```python
from build123d import *

# Parameters (mm, degrees)
CROQUIS1_W                 = 45
CROQUIS1_H                 = 45
SALIENTE_EXTRUIR1_DEPTH    = 300
CROQUIS4_W                 = 18
CROQUIS4_H                 = 34
CORTAR_EXTRUIR2_DEPTH      = 46
CROQUIS8_W                 = 35
CROQUIS8_H                 = 35
CORTAR_EXTRUIR3_DEPTH      = 301
CROQUIS9_W                 = 35
CROQUIS9_H                 = 21.174410022
CORTAR_EXTRUIR4_DEPTH      = 10
CROQUIS10_R                = 1
CORTAR_EXTRUIR5_DEPTH      = 10
CROQUIS11_W                = 45
CROQUIS11_H                = 26.387879272
CORTAR_EXTRUIR6_DEPTH      = 46
CROQUIS13_W                = 45
CROQUIS13_H                = 100
CORTAR_EXTRUIR7_DEPTH      = 23.5
CORTAR_EXTRUIR7_DEPTH_BACK = 23.5
CROQUIS14_W                = 55
CROQUIS14_H                = 55
SALIENTE_EXTRUIR2_DEPTH    = 5
CROQUIS16_R                = 1
CORTAR_EXTRUIR8_DEPTH      = 1
CORTAR_EXTRUIR8_DEPTH_BACK = 179.612120728
CROQUIS17_R                = 2.5
CROQUIS17_R_2              = 2.03
CROQUIS17_R_3              = 1.793308219
CORTAR_EXTRUIR9_DEPTH      = 6
CORTAR_EXTRUIR9_DEPTH_BACK = 51


with BuildPart() as part:
    # Croquis1 → Saliente-Extruir1 (new body)
    with BuildSketch(Plane(origin=(0, 0, 0), x_dir=(1, 0, 0), z_dir=(0, 1, 0))):
        Rectangle(CROQUIS1_W, CROQUIS1_H)
    extrude(amount=SALIENTE_EXTRUIR1_DEPTH)

    # Croquis4 → Cortar-Extruir2 (cut, through all)
    with BuildSketch(Plane.ZY.offset(22.5)):
        with Locations((13.5, 17)):
            Rectangle(CROQUIS4_W, CROQUIS4_H)
    extrude(amount=-CORTAR_EXTRUIR2_DEPTH, mode=Mode.SUBTRACT)

    # Croquis8 → Cortar-Extruir3 (cut, through all)
    with BuildSketch(Plane(origin=(0, 300, 0), x_dir=(1, 0, 0), z_dir=(0, 1, 0))):
        Rectangle(CROQUIS8_W, CROQUIS8_H)
    extrude(amount=-CORTAR_EXTRUIR3_DEPTH, mode=Mode.SUBTRACT)

    # Croquis9 → Cortar-Extruir4 (cut)
    with BuildSketch(Plane(origin=(0, 0, -22.5), x_dir=(-1, 0, 0), z_dir=(0, 0, -1))):
        with Locations((0, 260)):
            Rectangle(CROQUIS9_W, CROQUIS9_H)
    extrude(amount=-CORTAR_EXTRUIR4_DEPTH, mode=Mode.SUBTRACT)

    # Croquis10 → Cortar-Extruir5 (cut)
    with BuildSketch(Plane.XY.offset(22.5)):
        with Locations((0, 260)):
            Circle(CROQUIS10_R)
    extrude(amount=-CORTAR_EXTRUIR5_DEPTH, mode=Mode.SUBTRACT)

    # Croquis11 → Cortar-Extruir6 (cut, through all)
    with BuildSketch(Plane.XY.offset(22.5)):
        with Locations((0, 286.806060364)):
            Rectangle(CROQUIS11_W, CROQUIS11_H)
    extrude(amount=-CORTAR_EXTRUIR6_DEPTH, mode=Mode.SUBTRACT)

    # Croquis13 → Cortar-Extruir7 (cut, two sides)
    with BuildSketch(Plane(origin=(0, 0, 0), x_dir=(0, 0, -1), z_dir=(1, 0, 0))) as cortar_extruir7_sk:
        with Locations((0, 50)):
            Rectangle(CROQUIS13_W, CROQUIS13_H)
    extrude(amount=CORTAR_EXTRUIR7_DEPTH, mode=Mode.SUBTRACT)
    extrude(cortar_extruir7_sk.sketch, amount=-CORTAR_EXTRUIR7_DEPTH_BACK, mode=Mode.SUBTRACT)

    # Croquis14 → Saliente-Extruir2 (add)
    with BuildSketch(Plane.XZ.offset(-100)):
        Rectangle(CROQUIS14_W, CROQUIS14_H)
    extrude(amount=SALIENTE_EXTRUIR2_DEPTH)

    # Croquis16 → Cortar-Extruir8 (cut, two sides)
    with BuildSketch(Plane.XZ.offset(-95)) as cortar_extruir8_sk:
        with Locations((25, 25)):
            Circle(CROQUIS16_R)
        with Locations((-25, 25)):
            Circle(CROQUIS16_R)
        with Locations((-25, -25)):
            Circle(CROQUIS16_R)
        with Locations((25, -25)):
            Circle(CROQUIS16_R)
    extrude(amount=CORTAR_EXTRUIR8_DEPTH, mode=Mode.SUBTRACT)
    extrude(cortar_extruir8_sk.sketch, amount=-CORTAR_EXTRUIR8_DEPTH_BACK, mode=Mode.SUBTRACT)

    # Croquis17 → Cortar-Extruir9 (cut, two sides)
    with BuildSketch(Plane.XY.offset(22.5)) as cortar_extruir9_sk:
        with Locations((-10, 262.50260741)):
            Circle(CROQUIS17_R)
        with Locations((-10, 254.10260741)):
            Circle(CROQUIS17_R_2)
        with Locations((-10, 214.90260741)):
            Circle(CROQUIS17_R_3)
        with Locations((-10, 206.50260741)):
            Circle(CROQUIS17_R)
        with Locations((10, 262.50260741)):
            Circle(CROQUIS17_R)
        with Locations((10, 206.50260741)):
            Circle(CROQUIS17_R)
    extrude(amount=CORTAR_EXTRUIR9_DEPTH, mode=Mode.SUBTRACT)
    extrude(cortar_extruir9_sk.sketch, amount=-CORTAR_EXTRUIR9_DEPTH_BACK, mode=Mode.SUBTRACT)


solid = part.part
```
Here's how the part is built. I have some questions about the finished solid (model axes, mm). A direction names the side the tool comes from. Give positions to 0.01 mm unless a question says otherwise; leave off trailing zeros. Loops run counter-clockwise (first coordinate to the right, second up) from the corner with the lowest first, then second, coordinate; pieces in that order, holes last. Notation, with made-up numbers: M -2,-13 L 40,-13 A27 ccw 40,23 Z; hole C 46,65 d5. An arc over 180 degrees is marked long. Put each result on its own line as item: value. Start each with the question number.
(1) I need wall thicknesses on line 1 along Z through (x, y) = (25, 98); line 2 along X through (y, z) = (157, -16). Which ranges of each line are inside material? Lowest first, please. Write a range as [from, to].
(2) For faces 5 (the flat face through (0, 186, 22.5)), 6 (the flat face through (0, 186, -22.5)), 7 (the flat face through (-2, 100, 23)), which set-ups out of +Z, -Z, +X, -X, +Y, -Y let a thin tool reach every point of the face, with its end or its side?
(3) I want a section at C-C on z = 11. Please give me the cut outline in (x, y).
(4) I want a section at A-A on y = 202. Please give me the cut outline in (x, z), then the cut area to 3 significant figures.
(5) If we mould it in two halves opening along Y, with no side actions, what happens to faces 1 (the flat face through (0, 100, 0)), 2 (the cylindrical face through (-10.23, 216.68, -19.97)), 3 (the cylindrical face through (-10.54, 260.06, 20.04)), 4 (the flat face through (-22.5, 186, 0))? For each: +Y half, -Y half, draft (parallel to the pull), parting line (faces both ways), or undercut.
(6) I want a section at B-B on x = 4. Please give me the cut outline in (y, z), then the cut area to 3 significant figures.
(7) Will these pins go through, and if not, where does the flat tip stop? pin 1 Ø8 at (x, y) = (10, 262.5) entering from +Z; pin 2 Ø6 at (x, z) = (10.5, 7.5) entering from +Y; pin 3 Ø1 at (y, z) = (250.5, -4) entering from +X.
Answer block:
1. line 1: [-27.5, -26], [-24, 24], [26, 27.5]
1. line 2: [-22.5, -17.5], [17.5, 22.5]
2. face 5: +Z, +X, -X, +Y
2. face 6: -Z, +X, -X, +Y
2. face 7: +Y
3. outline: M -27.5,95 L 27.5,95 L 27.5,100 L 22.5,100 L 22.5,273.61 L 17.5,273.61 L 17.5,100 L -17.5,100 L -17.5,273.61 L -22.5,273.61 L -22.5,100 L -27.5,100 Z
4. outline: M -22.5,-22.5 L 22.5,-22.5 L 22.5,22.5 L -22.5,22.5 Z; hole M -17.5,-17.5 L 17.5,-17.5 L 17.5,17.5 L -17.5,17.5 Z
4. area: 800 mm^2
5. face 1: +Y half
5. face 2: undercut
5. face 3: undercut
5. face 4: draft
6. outline: M 95,-27.5 L 100,-27.5 L 100,-22.5 L 249.41,-22.5 L 249.41,-17.5 L 100,-17.5 L 100,17.5 L 273.61,17.5 L 273.61,22.5 L 100,22.5 L 100,27.5 L 95,27.5 Z; M 270.59,-22.5 L 273.61,-22.5 L 273.61,-17.5 L 270.59,-17.5 Z
6. area: 1,910 mm^2
7. pin 1: z = 22.5
7. pin 2: y = 100
7. pin 3: x = 22.5
